Design review of the part built by this model. Coordinates are the model's own, in mm. A direction names the side the tool comes from. Coordinates: 2 decimals unless noted, no trailing zeros. Loops run counter-clockwise (first coordinate to the right, second up) from the corner with the lowest first, then second, coordinate; pieces in that order, holes last.
Q1. Add section D-D on x = 5.25. Give the boundary of the cut face in (y, z).
Q2. Add section C-C on z = -7.75. Give the boundary of the cut face in (x, y).
Q3. Add section B-B on y = 2. Give the boundary of the cut face in (x, z).
Q4. Wall thickness on probe 1 along X at (y, z) = (6.75, -6); probe 2 along Y at (x, z) = (-3.5, -6); probe 3 along X at (y, z) = (5, 2.75): over which ranges is each line inside the solid? List them lowest first.
Q5. Add section A-A on z = 0. Give the boundary of the cut face in (x, y), and give its area (3 significant figures).
Q6. For P1, Ø4.5, axis at x = 4.5, z = -8.5, coming from the +Y side; P2, Ø2.5, axis at y = 4, z = -9, coming from the +X side; P3, Ø1.2, axis at x = 5, z = -8, coming from the -Y side, all flat-tipped, find the tip position at first contact; note any pin that passes through.
Q7. Machinability: for faces 5 (the face through (-4, 7.5, -7)), 6 (the face through (6.5, -5, -7)), 7 (the face through (2.5, 5, -7)), which of the approach directions +Z, -Z, +X, -X, +Y, -Y give a long, thin tool a straight path to every point of the face, cutting with its end or side? Answer none if there is none.
Q8. Draft analysis for pull direction Y (two halves, no side actions). For faces 1 (the face through (-6.5, -5, -7)), 2 (the face through (-5.5, 0, 1)), 3 (the face through (0, 5.5, 1)), 4 (the face through (-4, -7.5, -7)), state which applies: released by +Y, released by -Y, zero draft, split by the parting line, or undercut.
```python
from build123d import *

# Parameters (mm, degrees)
SKETCH1_W           = 15
SKETCH1_H           = 18
BOSS_EXTRUDE1_DEPTH = 3
SKETCH2_W           = 11
SKETCH2_H           = 11
CUT_EXTRUDE1_DEPTH  = 4
SKETCH4_W           = 4
SKETCH4_H           = 5
BOSS_EXTRUDE2_DEPTH = 8


with BuildPart() as part:
    # Sketch1 → Boss-Extrude1 (new, symmetric)
    with BuildSketch(Plane.XY):
        Rectangle(SKETCH1_W, SKETCH1_H)
    extrude(amount=BOSS_EXTRUDE1_DEPTH, both=True)

    # Sketch2 → Cut-Extrude1 (cut)
    with BuildSketch(Plane.XY.offset(3)):
        Rectangle(SKETCH2_W, SKETCH2_H)
    extrude(amount=-CUT_EXTRUDE1_DEPTH, mode=Mode.SUBTRACT)

    # Sketch4 → Boss-Extrude2 (add)
    with BuildSketch(Plane(origin=(0, 0, -3), x_dir=(-1, 0, 0), z_dir=(0, 0, -1))):
        with Locations((-4.5, 5)):
            Rectangle(SKETCH4_W, SKETCH4_H)
        with Locations((4.5, 5)):
            Rectangle(SKETCH4_W, SKETCH4_H)
        with Locations((4.5, -5)):
            Rectangle(SKETCH4_W, SKETCH4_H)
        with Locations((-4.5, -5)):
            Rectangle(SKETCH4_W, SKETCH4_H)
    extrude(amount=BOSS_EXTRUDE2_DEPTH)


solid = part.part
```
Entries:
1. outline: (-9, -3) - (-7.5, -3) - (-7.5, -11) - (-2.5, -11) - (-2.5, -3) - (2.5, -3) - (2.5, -11) - (7.5, -11) - (7.5, -3) - (9, -3) - (9, 3) - (5.5, 3) - (5.5, -1) - (-5.5, -1) - (-5.5, 3) - (-9, 3) - close
2. outline: (-6.5, -7.5) - (-2.5, -7.5) - (-2.5, -2.5) - (-6.5, -2.5) - close; (-6.5, 2.5) - (-2.5, 2.5) - (-2.5, 7.5) - (-6.5, 7.5) - close; (2.5, -7.5) - (6.5, -7.5) - (6.5, -2.5) - (2.5, -2.5) - close; (2.5, 2.5) - (6.5, 2.5) - (6.5, 7.5) - (2.5, 7.5) - close
3. outline: (-7.5, -3) - (7.5, -3) - (7.5, 3) - (5.5, 3) - (5.5, -1) - (-5.5, -1) - (-5.5, 3) - (-7.5, 3) - close
4. probe 1: x = -6.5 to -2.5, 2.5 to 6.5
4. probe 2: y = -7.5 to -2.5, 2.5 to 7.5
4. probe 3: x = -7.5 to -5.5, 5.5 to 7.5
5. outline: (-7.5, -9) - (7.5, -9) - (7.5, 9) - (-7.5, 9) - close; hole (-5.5, -5.5) - (5.5, -5.5) - (5.5, 5.5) - (-5.5, 5.5) - close
5. area: 149 mm2
6. P1: stops at y = 7.5
6. P2: stops at x = 6.5
6. P3: stops at y = -7.5
7. face 5: -Z, +X, -X, +Y
7. face 6: -Z, +X, +Y, -Y
7. face 7: -Z, +Y, -Y
8. face 1: zero draft
8. face 2: undercut
8. face 3: undercut
8. face 4: released by -Y
